Check sheet for the modelled part. Datum: model origin and axes. Units: mm. Face numbers are marked on the shaded views. Give positions to 0.01 mm unless a question says otherwise; leave off trailing zeros. Loops run counter-clockwise (first coordinate to the right, second up) from the corner with the lowest first, then second, coordinate; pieces in that order, holes last. Notation, with made-up numbers: (65.5, 84) -> (78.5, 84) arc R12 cw to (78.5, 94) -> close; hole circle Ø10 at (51.25, 7.5). An arc over 180 degrees is marked (long way). Write each question's results on one line, items separated by ' | '. Start each with the question number.
1. Cross-section at A-A on x = 6. Record the boundary of the cut face in (y, z), and give its area (3 significant figures).
2. Cross-section at B-B on z = -6. Record the boundary of the cut face in (x, y), and give its area (3 significant figures).
3. Material ranges on L1, parallel to Z at x = -5, y = 48.1 (3 decimals); L2, parallel to Y at x = 6.25, z = -5.25; L3, parallel to X at y = 20, z = 1.25, recorded low to high. Write a range as from..to.
4. Gauge pin test, flat ends, axial feed: pin 1 Ø5 at (y, z) = (15, 5.5) entering from -X; pin 2 Ø12 at (x, y) = (-2.5, 14.5) entering from +Z. Record the tip position at first contact, or that the pin passes through.
5. Mould release check, pull along Y, two halves, no side actions. Record for the marked faces 1, 2, 3 and 4: +Y half, -Y half, draft (parallel to the pull), parting line (faces both ways), or undercut.
6. Cross-section at C-C on y = 25.5. Record the boundary of the cut face in (x, z), and give its area (3 significant figures).
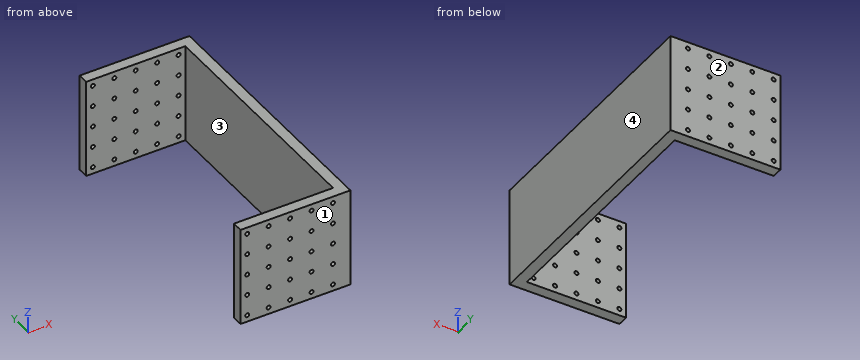
from build123d import *

# Parameters (mm, degrees)
SKETCH1_W           = 20.5
SKETCH1_H           = 18.5
BOSS_EXTRUDE1_DEPTH = 2
SKETCH2_W           = 2
SKETCH2_H           = 18.5
BOSS_EXTRUDE2_DEPTH = 45
SKETCH4_W           = 20.5
SKETCH4_H           = 18.5
BOSS_EXTRUDE3_DEPTH = 2
SKETCH3_R           = 0.375
CUT_EXTRUDE1_DEPTH  = 50


with BuildPart() as part:
    # Sketch1 → Boss-Extrude1 (new body)
    with BuildSketch(Plane(origin=(0, 0, 0), x_dir=(1, 0, 0), z_dir=(0, 1, 0))):
        Rectangle(SKETCH1_W, SKETCH1_H)
    extrude(amount=BOSS_EXTRUDE1_DEPTH)

    # Sketch2 → Boss-Extrude2 (add)
    with BuildSketch(Plane(origin=(0, 2, 0), x_dir=(1, 0, 0), z_dir=(0, 1, 0))):
        with Locations((9.25, 0)):
            Rectangle(SKETCH2_W, SKETCH2_H)
    extrude(amount=BOSS_EXTRUDE2_DEPTH)

    # Sketch4 → Boss-Extrude3 (add)
    with BuildSketch(Plane(origin=(0, 47, 0), x_dir=(1, 0, 0), z_dir=(0, 1, 0))):
        Rectangle(SKETCH4_W, SKETCH4_H)
    extrude(amount=BOSS_EXTRUDE3_DEPTH)

    # Sketch3 → Cut-Extrude1 (cut, through all)
    with BuildSketch(Plane.XZ):
        with Locations((-9, 8)):
            Circle(SKETCH3_R)
        with Locations((-5, 8)):
            Circle(SKETCH3_R)
        with Locations((-1, 8)):
            Circle(SKETCH3_R)
        with Locations((3, 8)):
            Circle(SKETCH3_R)
        with Locations((7, 8)):
            Circle(SKETCH3_R)
        with Locations((-5, 4)):
            Circle(SKETCH3_R)
        with Locations((-1, 4)):
            Circle(SKETCH3_R)
        with Locations((3, 4)):
            Circle(SKETCH3_R)
        with Locations((7, 4)):
            Circle(SKETCH3_R)
        with Locations((-5, 0)):
            Circle(SKETCH3_R)
        with Locations((-1, 0)):
            Circle(SKETCH3_R)
        with Locations((3, 0)):
            Circle(SKETCH3_R)
        with Locations((7, 0)):
            Circle(SKETCH3_R)
        with Locations((-5, -4)):
            Circle(SKETCH3_R)
        with Locations((-1, -4)):
            Circle(SKETCH3_R)
        with Locations((3, -4)):
            Circle(SKETCH3_R)
        with Locations((7, -4)):
            Circle(SKETCH3_R)
        with Locations((-5, -8)):
            Circle(SKETCH3_R)
        with Locations((-1, -8)):
            Circle(SKETCH3_R)
        with Locations((3, -8)):
            Circle(SKETCH3_R)
        with Locations((7, -8)):
            Circle(SKETCH3_R)
        with Locations((-5, -12)):
            Circle(SKETCH3_R)
        with Locations((-1, -12)):
            Circle(SKETCH3_R)
        with Locations((3, -12)):
            Circle(SKETCH3_R)
        with Locations((7, -12)):
            Circle(SKETCH3_R)
        with Locations((-9, 4)):
            Circle(SKETCH3_R)
        with Locations((-9, 0)):
            Circle(SKETCH3_R)
        with Locations((-9, -4)):
            Circle(SKETCH3_R)
        with Locations((-9, -8)):
            Circle(SKETCH3_R)
        with Locations((-9, -12)):
            Circle(SKETCH3_R)
    extrude(amount=-CUT_EXTRUDE1_DEPTH, mode=Mode.SUBTRACT)


solid = part.part
Geometry says:
1) outline: (0, -9.25) -> (2, -9.25) -> (2, 9.25) -> (0, 9.25) -> close; (47, -9.25) -> (49, -9.25) -> (49, 9.25) -> (47, 9.25) -> close | area: 74.0 mm^2
2) outline: (-10.25, 0) -> (10.25, 0) -> (10.25, 49) -> (-10.25, 49) -> (-10.25, 47) -> (8.25, 47) -> (8.25, 2) -> (-10.25, 2) -> close | area: 172 mm^2
3) L1: -9.25..-8.375, -7.625..-4.375, -3.625..-0.375, 0.375..3.625, 4.375..7.625, 8.375..9.25 | L2: 0..2, 47..49 | L3: 8.25..10.25
4) pin 1: x = 8.25 | pin 2: through
5) face 1: -Y half | face 2: +Y half | face 3: undercut | face 4: draft
6) outline: (8.25, -9.25) -> (10.25, -9.25) -> (10.25, 9.25) -> (8.25, 9.25) -> close | area: 37.0 mm^2
